Check sheet for the modelled part. Datum: model origin and axes. Units: mm. Face numbers are marked on the shaded views. A direction names the side the tool comes from. Round coordinates to 2 decimals unless told otherwise and drop trailing zeros. Write each loop counter-clockwise with the first axis right and the second up, starting at its lowest first coordinate (ties: lowest second). Pieces come first, ordered by that corner, then holes. Notation, with made-up numbers: (51, -23) -> (62, -23) arc R20 cw to (62, -19) -> close; hole circle Ø4 at (-28, 13.25). An arc over 180 degrees is marked (long way). One line per item, written item: value.
from build123d import *

# Parameters (mm, degrees)
SKETCH1_W           = 146.05
SKETCH1_H           = 90.678
SKETCH1_W_2         = 133.35
SKETCH1_H_2         = 77.978
BOSS_EXTRUDE1_DEPTH = 25.4
SKETCH2_W           = 60.325
SKETCH2_H           = 22.86
BOSS_EXTRUDE2_DEPTH = 6.35
CUT_EXTRUDE1_REACH  = 123.544
SKETCH6_W           = 53.975
SKETCH6_H           = 90.678
BOSS_EXTRUDE3_DEPTH = 44.45
CUT_EXTRUDE3_REACH  = 128.032
SKETCH8_W           = 41.275
SKETCH8_H           = 38.1


with BuildPart() as part:
    # Sketch1 → Boss-Extrude1 (new body)
    with BuildSketch(Plane.XY):
        Rectangle(SKETCH1_W, SKETCH1_H)
        Rectangle(SKETCH1_W_2, SKETCH1_H_2, mode=Mode.SUBTRACT)
    extrude(amount=BOSS_EXTRUDE1_DEPTH)

    # Sketch2 → Boss-Extrude2 (add)
    with BuildSketch(Plane(origin=(0, -45.339, 0), x_dir=(1, 0, 0), z_dir=(0, 1, 0))):
        Polygon((-40.513, -48.26), (-40.513, -25.4), (-73.025, -25.4), align=None)
        with Locations((-10.3505, -36.83)):
            Rectangle(SKETCH2_W, SKETCH2_H)
        Polygon((73.025, -25.4), (19.812, -25.4), (19.812, -48.26), align=None)
        Polygon((-73.025, -48.26), (-40.513, -48.26), (-73.025, -25.4), align=None)
        Polygon((73.025, -25.4), (19.812, -48.26), (73.025, -48.26), align=None)
    extrude(amount=BOSS_EXTRUDE2_DEPTH)

    # Sketch5 → Cut-Extrude1 (cut, up to next)
    with BuildSketch(Plane(origin=(0, -38.989, 0), x_dir=(1, 0, 0), z_dir=(0, 1, 0)), mode=Mode.PRIVATE) as cut_extrude1_sk1:
        with BuildLine():
            Line((-20.193, -38.735), (-20.193, -6.985))
            ThreePointArc((-20.193, -6.985), (-16.891, -3.683), (-13.589, -6.985))
            Line((-13.589, -6.985), (-13.589, -38.735))
            ThreePointArc((-13.589, -38.735), (-16.891, -42.037), (-20.193, -38.735))
        make_face()
    cut_extrude1_tool1 = extrude(cut_extrude1_sk1.sketch, amount=-CUT_EXTRUDE1_REACH, mode=Mode.PRIVATE) & part.part
    # Sketch5 → Cut-Extrude1 (cut, up to next)
    with BuildSketch(Plane(origin=(0, -38.989, 0), x_dir=(1, 0, 0), z_dir=(0, 1, 0)), mode=Mode.PRIVATE) as cut_extrude1_sk2:
        with BuildLine():
            Line((6.87705, -9.707286463), (6.87705, -41.457286463))
            ThreePointArc((6.87705, -41.457286463), (4.21005, -44.124286463), (1.54305, -41.457286463))
            Line((1.54305, -41.457286463), (1.54305, -9.707286463))
            ThreePointArc((1.54305, -9.707286463), (4.21005, -7.040286463), (6.87705, -9.707286463))
        make_face()
    cut_extrude1_tool2 = extrude(cut_extrude1_sk2.sketch, amount=-CUT_EXTRUDE1_REACH, mode=Mode.PRIVATE) & part.part
    # Sketch5 → Cut-Extrude1 (cut, up to next)
    with BuildSketch(Plane(origin=(0, -38.989, 0), x_dir=(1, 0, 0), z_dir=(0, 1, 0)), mode=Mode.PRIVATE) as cut_extrude1_sk3:
        with BuildLine():
            Line((-40.65905, -9.707286463), (-40.65905, -41.457286463))
            ThreePointArc((-40.65905, -41.457286463), (-37.99205, -44.124286463), (-35.32505, -41.457286463))
            Line((-35.32505, -41.457286463), (-35.32505, -9.707286463))
            ThreePointArc((-35.32505, -9.707286463), (-37.99205, -7.040286463), (-40.65905, -9.707286463))
        make_face()
    cut_extrude1_tool3 = extrude(cut_extrude1_sk3.sketch, amount=-CUT_EXTRUDE1_REACH, mode=Mode.PRIVATE) & part.part
    add(cut_extrude1_tool1.solids().sort_by_distance((-16.891, -38.989, 22.86))[0], mode=Mode.SUBTRACT)
    add(cut_extrude1_tool2.solids().sort_by_distance((4.21005, -38.989, 25.582286))[0], mode=Mode.SUBTRACT)
    add(cut_extrude1_tool3.solids().sort_by_distance((-37.99205, -38.989, 25.582286))[0], mode=Mode.SUBTRACT)

    # Sketch6 → Boss-Extrude3 (add)
    with BuildSketch(Plane(origin=(0, 0, 0), x_dir=(-1, 0, 0), z_dir=(0, 0, -1))):
        with Locations((-46.0375, 0)):
            Rectangle(SKETCH6_W, SKETCH6_H)
    extrude(amount=BOSS_EXTRUDE3_DEPTH)

    # Sketch8 → Cut-Extrude3 (cut, up to next)
    with BuildSketch(Plane(origin=(0, 45.339, 0), x_dir=(1, 0, 0), z_dir=(0, 1, 0)), mode=Mode.PRIVATE) as cut_extrude3_sk1:
        with Locations((46.0375, 19.05)):
            Rectangle(SKETCH8_W, SKETCH8_H)
    cut_extrude3_tool1 = extrude(cut_extrude3_sk1.sketch, amount=-CUT_EXTRUDE3_REACH, mode=Mode.PRIVATE) & part.part
    add(cut_extrude3_tool1.solids().sort_by_distance((46.0375, 45.339, -19.05))[0], mode=Mode.SUBTRACT)


solid = part.part
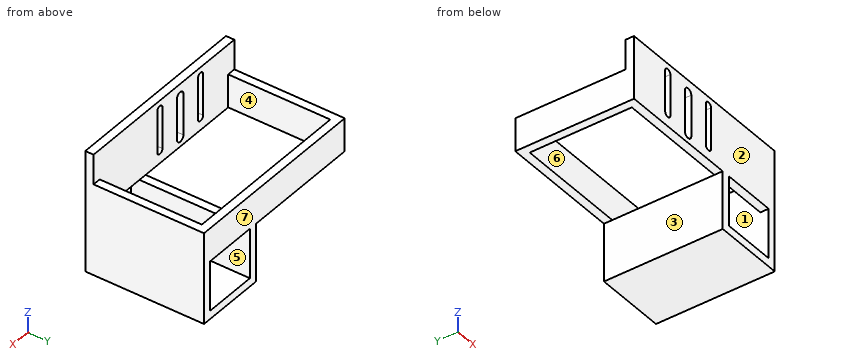
Item 1: Sectioned sample at A-A (x = 57.5). Enter the section's corners in (y, z), then the cut area to 3 significant figures.
Result set:
outline: (-45.34, -44.45) -> (45.34, -44.45) -> (45.34, -38.1) -> (-45.34, -38.1) -> close; (-45.34, 0) -> (-38.99, 0) -> (-38.99, 48.26) -> (-45.34, 48.26) -> close; (38.99, 0) -> (45.34, 0) -> (45.34, 25.4) -> (38.99, 25.4) -> close
area: 1,040 mm^2
Item 2: Depth check by flat-ended pin: pin 1 (5 mm diameter, centred on x = 21.5, y = 8, fed in from +Z); pin 2 (3 mm diameter, centred on y = -23, z = -20.5, fed in from -X); pin 3 (8 mm diameter, centred on x = -19.5, y = -33.5, fed in from +Z). Enter the tip coordinate at first touch or a pass-through.
Result set:
pin 1: z = 0
pin 2: x = 19.05
pin 3: through
Item 3: Release check for a two-part mould opening along Y. For the marked faces 1, 2 and 3 record: pulls with the +Y half, pulls with the -Y half, needs draft (parallel to the pull), parting line crosses it, or undercut.
Result set:
face 1: undercut
face 2: pulls with the -Y half
face 3: needs draft
Item 4: Sectioned sample at B-B (z = -4). Enter the section's corners in (x, y) (3 decimals), then the cut area to 3 significant figures.
Result set:
outline: (19.05, -45.339) -> (25.4, -45.339) -> (25.4, 45.339) -> (19.05, 45.339) -> close; (66.675, -45.339) -> (73.025, -45.339) -> (73.025, 45.339) -> (66.675, 45.339) -> close
area: 1,150 mm^2
Item 5: Material ranges on line 1 along X through (y, z) = (-12, -1.5) (3 decimals); line 2 along Y through (x, z) = (15, 11); line 3 along Y through (x, z) = (10.5, 36.5), recorded low to high.
Result set:
line 1: 19.05 to 25.4, 66.675 to 73.025
line 2: -45.34 to -38.99, 38.99 to 45.34
line 3: -45.34 to -38.99
Item 6: Tool access check on the marked faces 4, 5, 6 and 7. Record the directions out of +Z, -Z, +X, -X, +Y, -Y that give a thin tool (end or side, any length) a straight path to the whole face; none if there is none.
Result set:
face 4: +Z, -Z
face 5: +Y, -Y
face 6: +Z
face 7: +Z, -Z, +X, -X, +Y
Item 7: Sectioned sample at D-D (x = -44.5). Enter the section's corners in (y, z), then the cut area to 3 significant figures.
Result set:
outline: (-45.34, 0) -> (-38.99, 0) -> (-38.99, 48.26) -> (-45.34, 48.26) -> close; (38.99, 0) -> (45.34, 0) -> (45.34, 25.4) -> (38.99, 25.4) -> close
area: 468 mm^2
Item 8: Sectioned sample at C-C (y = 29.5). Enter the section's corners in (x, z) (3 decimals).
Result set:
outline: (-73.025, 0) -> (-66.675, 0) -> (-66.675, 25.4) -> (-73.025, 25.4) -> close; (19.05, -44.45) -> (73.025, -44.45) -> (73.025, 25.4) -> (66.675, 25.4) -> (66.675, -38.1) -> (25.4, -38.1) -> (25.4, 0) -> (19.05, 0) -> close
